from build123d import *

# Parameters (mm, degrees)
SKETCH_R     = 5
PAD_DEPTH    = 1.6
PAD001_DEPTH = 13


with BuildPart() as part:
    # Sketch → Pad (new body)
    with BuildSketch(Plane.XY):
        with Locations((-0.010221, -0.048828)):
            Circle(SKETCH_R)
        Polygon((2.165064, -1.25), (2.165064, 1.25), (0, 2.5), (-2.165064, 1.25), (-2.165064, -1.25), (0, -2.5), align=None, mode=Mode.SUBTRACT)
    extrude(amount=PAD_DEPTH)

    # Sketch001 → Pad001 (new body)
    with BuildSketch(Plane.XY.offset(1.6)):
        Polygon((3.117691, -1.8), (3.117691, 1.8), (0, 3.6), (-3.117691, 1.8), (-3.117691, -1.8), (0, -3.6), align=None)
        Polygon((2.165064, -1.25), (2.165064, 1.25), (0, 2.5), (-2.165064, 1.25), (-2.165064, -1.25), (0, -2.5), align=None, mode=Mode.SUBTRACT)
    extrude(amount=PAD001_DEPTH)


solid = part.part
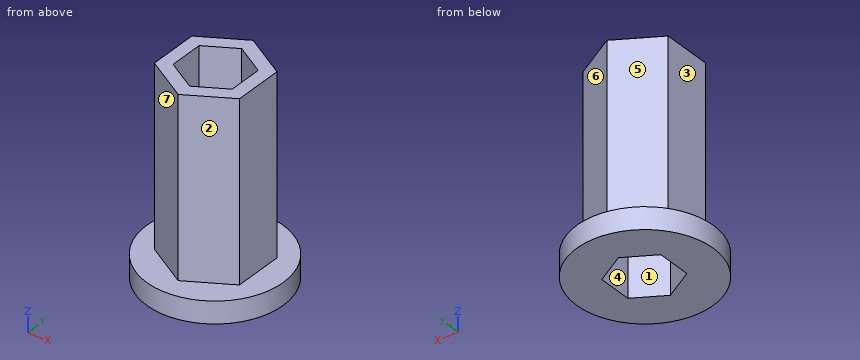
Verification items for the finished model (mm, model axes). Face numbers are marked on the shaded views. A direction names the side the tool comes from. Coordinates: 2 decimals unless noted, no trailing zeros. Order: outer loops, then holes, each group sorted by start corner. A loop starts at its lowest first (then second) coordinate and runs counter-clockwise, first axis right, second up. Notation, with made-up numbers: (-30, -21) -> (25, -21) arc R16 ccw to (25, -6) -> close; hole circle Ø2 at (36.5, 17). An arc over 180 degrees is marked (long way). Put each result on its own line as item: value. Start each with the question number.
1. Mould release check, pull along Y, two halves, no side actions. Record for the marked faces 1, 2 and 3: released by +Y, released by -Y, zero draft, split by the parting line, or undercut.
2. Cross-section at B-B, the plane y = -0.5. Record the boundary of the cut face in (x, z).
3. Go/stop test with flat-tipped pins: pin 1 Ø0.8 at (y, z) = (0.5, 8.5) entering from +X; pin 2 Ø3 at (y, z) = (-0.5, 11) entering from -X; pin 3 Ø5 at (x, z) = (2, 10.5) entering from +Y. Record where each tip stops, or that it passes through.
4. Material ranges on L1, parallel to X at y = 0.5, z = 3.75; L2, parallel to Z at x = -1.5, y = -4.5; L3, parallel to Y at x = 0.5, z = 9.75, recorded low to high. Write a range as [from, to].
5. Cross-section at C-C, the plane x = -0.25. Record the boundary of the cut face in (y, z), then the cut area to 3 significant figures.
6. Access from +Z, -Z, +X, -X, +Y, -Y to the whole of each face (thin tool, end or side, straight path). Record for the marked faces 4, 5, 6 and 7.
7. Cross-section at D-D, the plane x = 2.75. Record the boundary of the cut face in (y, z).
8. Cross-section at A-A, the plane z = 7.5. Record the boundary of the cut face in (x, y), then the cut area to 3 significant figures.
Computed:
1. face 1: undercut
1. face 2: released by -Y
1. face 3: zero draft
2. outline: (-4.99, 0) -> (-2.17, 0) -> (-2.17, 14.6) -> (-3.12, 14.6) -> (-3.12, 1.6) -> (-4.99, 1.6) -> close; (2.17, 0) -> (4.97, 0) -> (4.97, 1.6) -> (3.12, 1.6) -> (3.12, 14.6) -> (2.17, 14.6) -> close
3. pin 1: x = 3.12
3. pin 2: x = -3.12
3. pin 3: y = 3.6
4. L1: [-3.12, -2.17], [2.17, 3.12]
4. L2: [0, 1.6]
4. L3: [-3.31, -2.21], [2.21, 3.31]
5. outline: (-5.04, 0) -> (-2.36, 0) -> (-2.36, 14.6) -> (-3.46, 14.6) -> (-3.46, 1.6) -> (-5.04, 1.6) -> close; (2.36, 0) -> (4.95, 0) -> (4.95, 1.6) -> (3.46, 1.6) -> (3.46, 14.6) -> (2.36, 14.6) -> close
5. area: 37.0 mm2
6. face 4: +Z, -Z
6. face 5: +Z, -X, +Y
6. face 6: +Z, +X, +Y
6. face 7: +Z, -X, -Y
7. outline: (-4.22, 0) -> (4.12, 0) -> (4.12, 1.6) -> (2.01, 1.6) -> (2.01, 14.6) -> (-2.01, 14.6) -> (-2.01, 1.6) -> (-4.22, 1.6) -> close
8. outline: (-3.12, -1.8) -> (0, -3.6) -> (3.12, -1.8) -> (3.12, 1.8) -> (0, 3.6) -> (-3.12, 1.8) -> close; hole (-2.17, -1.25) -> (0, -2.5) -> (2.17, -1.25) -> (2.17, 1.25) -> (0, 2.5) -> (-2.17, 1.25) -> close
8. area: 17.4 mm2
